```python
from build123d import *

# Parameters (mm, degrees)
F1_DEPTH = 4.7625
F2_DEPTH = 7.9375
F3_SCALE = 0.75
F4_R     = 1.5875
F5_R     = 1.5875


with BuildPart() as f1:
    # F0 (on Top) → F1 (new body)
    with BuildSketch(Plane.XY):
        Polygon((47.0052342629, 0), (27.7066360927, 0), (25.7264233393, -7.5556741843), (37.7154810129, -7.5556741843), (35.7815611768, -14.9347137119), (23.7925035033, -14.9347137119), (21.7058496291, -22.8965232611), (33.6949073026, -22.8965232611), (30.1152669523, -36.5549527094), (15.6817594308, -43.6786170032), (13.1379523639, -53.3847343652), (35.9669688721, -42.117462739), align=None)
    extrude(amount=F1_DEPTH)



with BuildPart() as f1b:
    # F0 (on Top) → F1, piece 2 (new body)
    with BuildSketch(Plane.XY):
        Polygon((18.1816360927, 0), (0, 0), (-6.0106108367, -22.9340090122), (5.9414930498, -22.9340090122), (2.3059199107, -36.8058548863), (-12.1803115812, -44.5428210678), (-14.6133578163, -53.8263208316), (7.1163145289, -42.2206979224), align=None)
        Polygon((2.1785185584, -15.2999901774), (4.1821230904, -7.6550626248), (9.9458431257, -7.6550626248), (7.9422385937, -15.2999901774), align=None, mode=Mode.SUBTRACT)
    extrude(amount=F1_DEPTH)


with BuildPart() as f1c:
    # F0 (on Top) → F1, piece 3 (new body)
    with BuildSketch(Plane.XY):
        Polygon((-9.525, 0), (-29.1394729799, 0), (-31.1543771622, -7.6880423522), (-17.9473215339, -7.6880423522), (-19.9244964638, -15.2321254565), (-33.1315520921, -15.2321254565), (-40.2081700043, -42.2335772864), (-22.8844385775, -53.6695948649), (-20.7011714692, -44.6316399521), (-32.4044549927, -36.9058819843), (-28.7720391484, -23.0460830432), (-15.5649835201, -23.0460830432), align=None)
    extrude(amount=F1_DEPTH)


with BuildPart() as f1_1:
    add(f1.part)

    add(f1b.part)  # F2 merges F1b

    add(f1c.part)  # F2 merges F1c
    # F0 (on Top) → F2 (join)
    with BuildSketch(Plane.XY):
        with BuildLine():
            ThreePointArc((-30.3934413824, 4.7752), (-34.2728688515, 3.4523803739), (-36.5359867792, 0.0350559091))
            Line((-36.5359867792, 0.0350559091), (-49.8497964294, -50.7649440909))
            ThreePointArc((-49.8497964294, -50.7649440909), (-48.7344314064, -56.2542274692), (-43.7072510326, -58.7248))
            Line((-43.7072510326, -58.7248), (34.1189475279, -58.7248))
            ThreePointArc((34.1189475279, -58.7248), (37.9983749971, -57.4019803739), (40.2614929247, -53.9846559091))
            Line((40.2614929247, -53.9846559091), (53.5753025749, -3.1846559091))
            ThreePointArc((53.5753025749, -3.1846559091), (52.4599375519, 2.3046274692), (47.4327571781, 4.7752))
            Line((47.4327571781, 4.7752), (-30.3934413824, 4.7752))
        make_face()
        Polygon((-31.1543771622, -7.6880423522), (-29.1394729799, 0), (-9.525, 0), (-15.5649835201, -23.0460830432), (-28.7720391484, -23.0460830432), (-32.4044549927, -36.9058819843), (-20.7011714692, -44.6316399521), (-22.8844385775, -53.6695948649), (-40.2081700043, -42.2335772864), (-33.1315520921, -15.2321254565), (-19.9244964638, -15.2321254565), (-17.9473215339, -7.6880423522), align=None, mode=Mode.SUBTRACT)
        Polygon((-6.0106108367, -22.9340090122), (0, 0), (18.1816360927, 0), (7.1163145289, -42.2206979224), (-14.6133578163, -53.8263208316), (-12.1803115812, -44.5428210678), (2.3059199107, -36.8058548863), (5.9414930498, -22.9340090122), align=None, mode=Mode.SUBTRACT)
        Polygon((25.7264233393, -7.5556741843), (27.7066360927, 0), (47.0052342629, 0), (35.9669688721, -42.117462739), (13.1379523639, -53.3847343652), (15.6817594308, -43.6786170032), (30.1152669523, -36.5549527094), (33.6949073026, -22.8965232611), (21.7058496291, -22.8965232611), (23.7925035033, -14.9347137119), (35.7815611768, -14.9347137119), (37.7154810129, -7.5556741843), align=None, mode=Mode.SUBTRACT)
        Polygon((18.1816360927, 0), (0, 0), (-6.0106108367, -22.9340090122), (5.9414930498, -22.9340090122), (2.3059199107, -36.8058548863), (-12.1803115812, -44.5428210678), (-14.6133578163, -53.8263208316), (7.1163145289, -42.2206979224), align=None)
        Polygon((2.1785185584, -15.2999901774), (4.1821230904, -7.6550626248), (9.9458431257, -7.6550626248), (7.9422385937, -15.2999901774), align=None, mode=Mode.SUBTRACT)
        Polygon((47.0052342629, 0), (27.7066360927, 0), (25.7264233393, -7.5556741843), (37.7154810129, -7.5556741843), (35.7815611768, -14.9347137119), (23.7925035033, -14.9347137119), (21.7058496291, -22.8965232611), (33.6949073026, -22.8965232611), (30.1152669523, -36.5549527094), (15.6817594308, -43.6786170032), (13.1379523639, -53.3847343652), (35.9669688721, -42.117462739), align=None)
        Polygon((-9.525, 0), (-29.1394729799, 0), (-31.1543771622, -7.6880423522), (-17.9473215339, -7.6880423522), (-19.9244964638, -15.2321254565), (-33.1315520921, -15.2321254565), (-40.2081700043, -42.2335772864), (-22.8844385775, -53.6695948649), (-20.7011714692, -44.6316399521), (-32.4044549927, -36.9058819843), (-28.7720391484, -23.0460830432), (-15.5649835201, -23.0460830432), align=None)
        Polygon((9.9458431257, -7.6550626248), (4.1821230904, -7.6550626248), (2.1785185584, -15.2999901774), (7.9422385937, -15.2999901774), align=None)
    extrude(amount=-F2_DEPTH)


with BuildPart() as f1_2:
    # F3: moved
    add(f1_1.part.scale(F3_SCALE))

    # F4
    f4_edges = [f1_2.edges().sort_by_distance(p)[0] for p in [
        (-21.854605, 0, 1.785938),
        (-23.365783, -5.766032, 1.785938),
        (-13.460491, -5.766032, 1.785938),
        (-14.943372, -11.424094, 1.785938),
        (-24.848664, -11.424094, 1.785938),
        (-30.156128, -31.675183, 1.785938),
        (-17.163329, -40.252196, 1.785938),
        (-15.525879, -33.47373, 1.785938),
        (-21.579029, -17.284562, 1.785938),
        (-11.673738, -17.284562, 1.785938),
        (-4.507958, -17.200507, 1.785938),
        (4.45612, -17.200507, 1.785938),
        (1.72944, -27.604391, 1.785938),
        (-9.135234, -33.407116, 1.785938),
        (-10.960018, -40.369741, 1.785938),
        (5.337236, -31.665523, 1.785938),
        (13.636227, 0, 1.785938),
        (0, 0, 1.785938),
        (3.136592, -5.741297, 1.785938),
        (1.633889, -11.474993, 1.785938),
        (7.459382, -5.741297, 1.785938),
        (5.956679, -11.474993, 1.785938),
        (-7.14375, 0, 1.785938),
    ]]
    fillet(f4_edges, radius=F4_R)

    # F5
    f5_edges = [f1_2.edges().sort_by_distance(p)[0] for p in [
        (28.286611, -5.666756, 1.785938),
        (19.294818, -5.666756, 1.785938),
        (20.779977, 0, 1.785938),
        (17.844378, -11.201035, 1.785938),
        (16.279387, -17.172392, 1.785938),
        (25.27118, -17.172392, 1.785938),
        (11.76132, -32.758963, 1.785938),
        (9.853464, -40.038551, 1.785938),
        (26.975227, -31.588097, 1.785938),
        (22.58645, -27.416215, 1.785938),
        (26.836171, -11.201035, 1.785938),
        (35.253926, 0, 1.785938),
    ]]
    fillet(f5_edges, radius=F5_R)


solid = f1_2.part
```
Input: part model. Units: mm. Frame: model coordinates. A direction names the side the tool comes from. Round coordinates to 2 decimals unless told otherwise and drop trailing zeros. Loops run counter-clockwise (first coordinate to the right, second up) from the corner with the lowest first, then second, coordinate; pieces in that order, holes last. Notation, with made-up numbers: M -6,28 L 15,28 A34 cw 15,60 Z; hole C 28.5,-29.75 d11. An arc over 180 degrees is marked long. Answer in a Markdown table with one row per item. Add a question column.
1. Section D-D (y = -22). Output: boundary loops of the cut face in (x, z).
2. Contact query for flat-ended pins moving along their axis: pin 1 (4 mm diameter, centred on x = 20, z = 1.5, fed in from -Y); pin 2 (1 mm diameter, centred on y = -15.5, z = 1.5, fed in from +X); pin 3 (1.8 mm diameter, centred on x = -18.5, z = 2.5, fed in from +Y); pin 4 (4 mm diameter, centred on y = -23, z = -2.5, fed in from +X). Output: stop coordinate, or through.
3. Set-up query: faces 1 (the face through (-29.82, -31.53, 1.81)), 2 (the face through (24.458, -17.774, 1.811)), 3 (the face through (19.56, -35.25, 1.76)), 4 (the face through (0.27, -0.32, 1.81)), 5 (the face through (-21.588, -0.322, 1.811)). Return all of +Z, -Z, +X, -X, +Y, -Y with unobstructed straight access to the full face (end or side cutting, diameter ignored); none if empty.
4. Mould query, pull axis X, two halves, no side actions, for faces 6 (the face through (28.46, -43.08, -2.93)), 7 (the face through (-16.216, -36.33, 1.761)), 8 (the face through (28, 0, 2)). Classes: released by +X, released by -X, zero draft, split by the parting line, or undercut.
5. Section A-A (z = -5). Output: boundary loops of the cut face in (x, y) (1 decimal), and give its area (3 significant figures).
6. Section C-C (x = 15.5). Output: boundary loops of the cut face in (y, z).
7. Section B-B (y = -29). Output: boundary loops of the cut face in (x, z) (3 decimals).
8. Ray query, probe 1 along X at (y, z) = (-28, 1.5); probe 2 along X at (y, z) = (-19.5, 2.5); probe 3 along Z at (x, y) = (34, -7). Return the intervals inside material, ascending.
Values follow:
| question | item | result |
|---|---|---|
| 1 | outline | M -33.17,-5.95 L 35.04,-5.95 L 35.04,0 L 29.49,0 L 29.49,3.57 L 24.01,3.57 L 24.01,0 L 7.87,0 L 7.87,3.57 L 3.2,3.57 L 3.2,0 L -22.81,0 L -22.81,3.57 L -27.62,3.57 L -27.62,0 L -33.17,0 Z |
| 2 | pin 1 | y = -44.04 |
| 2 | pin 2 | x = 31.32 |
| 2 | pin 3 | y = 0 |
| 2 | pin 4 | x = 35.3 |
| 3 | face 1 | +Z, -X |
| 3 | face 2 | +Z |
| 3 | face 3 | +Z, +X, -Y |
| 3 | face 4 | +Z, +Y |
| 3 | face 5 | +Z, -X, +Y |
| 4 | face 6 | released by +X |
| 4 | face 7 | undercut |
| 4 | face 8 | zero draft |
| 5 | outline | M -37.4,-38.1 A4.8 ccw -32.8,-44 L 25.6,-44 A4.8 ccw 30.2,-40.5 L 40.2,-2.4 A4.8 ccw 35.6,3.6 L -22.8,3.6 A4.8 ccw -27.4,0 Z |
| 5 | area | 3,230 mm^2 |
| 6 | outline | M -44.04,-5.95 L 3.58,-5.95 L 3.58,0 L -30.91,0 L -30.91,3.57 L -37.25,3.57 L -37.25,0 L -44.04,0 Z |
| 7 | outline | M -35.009,-5.953 L 33.207,-5.953 L 33.207,0 L 27.654,0 L 27.654,3.572 L 19.377,3.572 L 19.377,0 L 6.036,0 L 6.036,3.572 L -0.884,3.572 L -0.884,0 L -22.303,0 L -22.303,3.572 L -29.455,3.572 L -29.455,0 L -35.009,0 Z |
| 8 | probe 1 | -29.19 to -23.82, 0.99 to 6.3, 21.4 to 27.92 |
| 8 | probe 2 | -26.97 to -22.16, 3.85 to 8.53, 24.66 to 30.14 |
| 8 | probe 3 | -5.95 to 0 |
